Source: CAD feature listing. Evaluate the final solid. Frame: model axes, mm. Round coordinates to 2 decimals unless told otherwise and drop trailing zeros. Loops run counter-clockwise (first coordinate to the right, second up) from the corner with the lowest first, then second, coordinate; pieces in that order, holes last. Notation, with made-up numbers: M 61.5,76.5 L 69.5,76.5 A17 cw 69.5,109.5 Z; hole C 32.5,22 d6. An arc over 180 degrees is marked long. Answer as a JSON object with one key per item and string values.
from build123d import *

# Parameters (mm, degrees)
SKETCH1_R           = 64
SKETCH1_R_2         = 62.5
BOSS_EXTRUDE1_DEPTH = 685
SKETCH2_W           = 7
SKETCH2_H           = 380
CUT_EXTRUDE1_DEPTH  = 75
CIRPATTERN1_COUNT   = 4
SKETCH3_R           = 1.5
CUT_EXTRUDE2_DEPTH  = 691.953688752


with BuildPart() as part:
    # Sketch1 → Boss-Extrude1 (new, symmetric)
    with BuildSketch(Plane.XY):
        Circle(SKETCH1_R)
        Circle(SKETCH1_R_2, mode=Mode.SUBTRACT)
    extrude(amount=BOSS_EXTRUDE1_DEPTH, both=True)

    # Sketch2 → Cut-Extrude1 (cut, symmetric)
    with BuildSketch(Plane(origin=(0, 0, 0), x_dir=(1, 0, 0), z_dir=(0, 1, 0))):
        with Locations((0, -480)):
            Rectangle(SKETCH2_W, SKETCH2_H)
    cut_extrude1 = extrude(amount=CUT_EXTRUDE1_DEPTH, both=True, mode=Mode.SUBTRACT)

    # CirPattern1: Cut-Extrude1 ×4 about axis
    cirpattern1_axis = Axis((0, 0, 685), (0, 0, 1))
    for i in range(1, CIRPATTERN1_COUNT):
        add(cut_extrude1.rotate(cirpattern1_axis, i * 360 / CIRPATTERN1_COUNT), mode=Mode.SUBTRACT)

    # Sketch3 → Cut-Extrude2 (cut, through all)
    with BuildSketch(Plane(origin=(0, 0, 0), x_dir=(1, 0, 0), z_dir=(0, 1, 0))):
        with Locations(Location((0, 645, 0), (0, 0, 90))):
            Circle(SKETCH3_R)
    extrude(amount=CUT_EXTRUDE2_DEPTH, mode=Mode.SUBTRACT)


solid = part.part
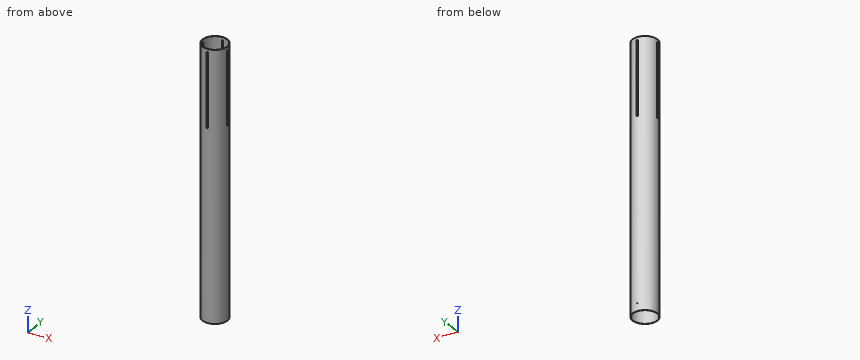
Item 1: Line query: probe 1 along Y at (x, z) = (0, -202.5); probe 2 along Y at (x, z) = (26, 0.5); probe 3 along X at (y, z) = (-27.5, -609). Output: solid intervals per line, ascending. Write a range as from..to.
Answer sheet:
{"probe 1": "y = -64..-62.5, 62.5..64", "probe 2": "y = -58.48..-56.84, 56.84..58.48", "probe 3": "x = -57.79..-56.12, 56.12..57.79"}
Item 2: Section C-C on x = -17. Return the cut outline in (y, z), then the cut area to 3 significant figures.
Answer sheet:
{"outline": "M -61.7,-685 L -60.14,-685 L -60.14,685 L -61.7,685 Z; M 60.14,-685 L 61.7,-685 L 61.7,685 L 60.14,685 Z", "area": "4,270 mm²"}
Item 3: Section A-A on z = 372.5. Return the cut outline in (x, y), then the cut area to 3 significant figures.
Answer sheet:
{"outline": "M -63.9,-3.5 A64 ccw -3.5,-63.9 L -3.5,-62.4 A62.5 cw -62.4,-3.5 Z; M -63.9,3.5 L -62.4,3.5 A62.5 cw -3.5,62.4 L -3.5,63.9 A64 ccw Z; M 3.5,-63.9 A64 ccw 63.9,-3.5 L 62.4,-3.5 A62.5 cw 3.5,-62.4 Z; M 3.5,62.4 A62.5 cw 62.4,3.5 L 63.9,3.5 A64 ccw 3.5,63.9 Z", "area": "554 mm²"}
Item 4: Section D-D on z = 46.5. Return the cut outline in (x, y).
Answer sheet:
{"outline": "C 0,0 d128; hole C 0,0 d125"}
Item 5: Contact query for flat-ended pins moving along their axis: pin 1 Ø5 at (y, z) = (-22, -235) entering from +X; pin 2 Ø1 at (y, z) = (-27, -520.5) entering from -X; pin 3 Ø1.5 at (x, z) = (-7, 74) entering from -Y; pin 4 Ø10 at (y, z) = (-2.5, -250) entering from -X. Output: stop coordinate, or through.
Answer sheet:
{"pin 1": "stops at x = 60.96", "pin 2": "stops at x = -58.26", "pin 3": "stops at y = -63.69", "pin 4": "stops at x = -64"}
Item 6: Section B-B on y = -29. Return the cut outline in (x, z), then the cut area to 3 significant figures.
Answer sheet:
{"outline": "M -57.05,-685 L -55.36,-685 L -55.36,685 L -57.05,685 Z; M 55.36,-685 L 57.05,-685 L 57.05,685 L 55.36,685 Z", "area": "4,620 mm²"}
